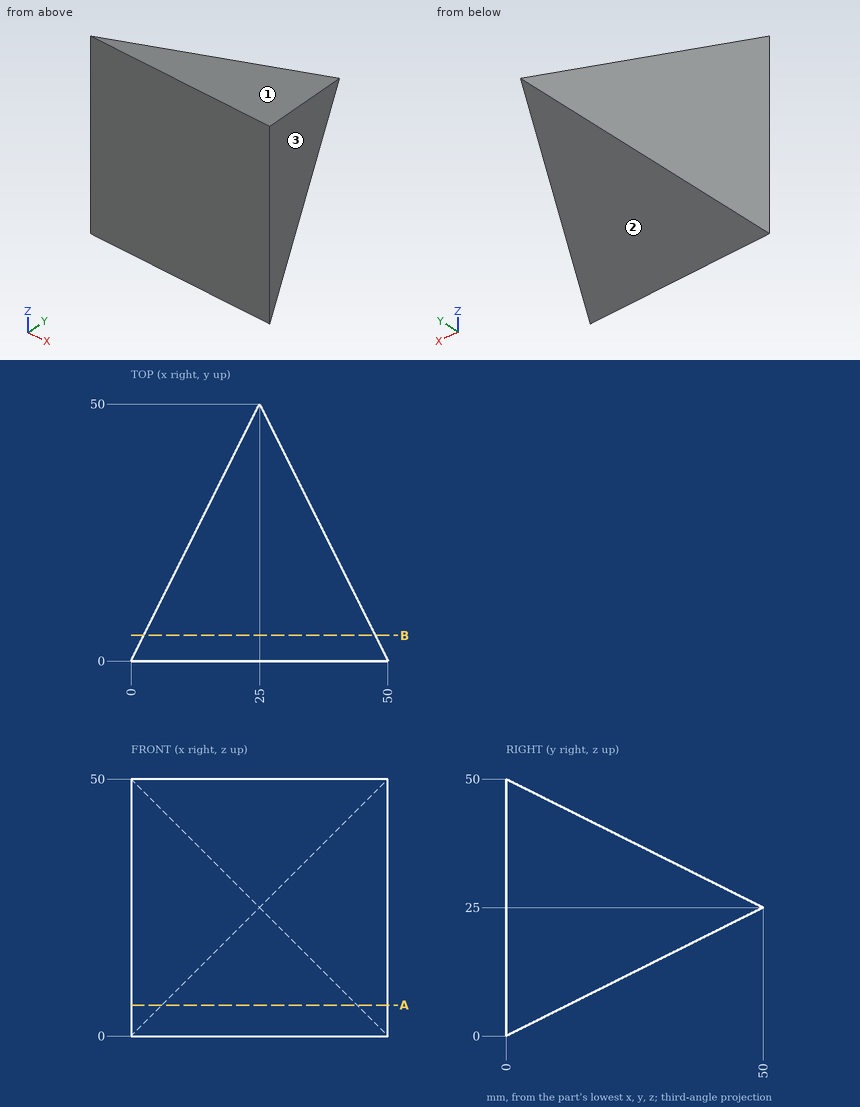
Study the drawing (mm; zero at the part's minimum x, y, z) and answer. Coordinates: 2 decimals unless noted, no trailing zeros. Loops run counter-clockwise (first coordinate to the right, second up) from the corner with the lowest first, then second, coordinate; pieces in that order, holes last. Notation, with made-up numbers: (67, 0) -> (113, 0) arc R29 ccw to (113, 37) -> close; hole circle Ø6 at (24.25, 59.25). An arc over 180 degrees is marked (long way). Write item = value, one per line. Start each with the question number.
1) The mould has two halves that part along Z. Classify the marked faces 1, 2 and 3: pulls with the +Z half, pulls with the -Z half, needs draft (parallel to the pull), parting line crosses it, or undercut.
2) Given P1, Ø1, axis at y = 25, z = 13.5, coming from the -X side; P2, Ø10, axis at y = 17.5, z = 34.5, coming from the -X side; P3, Ø4, axis at y = 7, z = 20.5, coming from the +X side, each flat-ended and moving along its own axis, determine where each tip first touches the part or whether it passes through.
3) Find the intervals of material crossed by L1, parallel to X at y = 45.5, z = 27; L2, parallel to Y at x = 38, z = 42; L3, parallel to Y at x = 47, z = 31.5, in increasing order. Write a range as from..to.
4) The part is cut by section B-B, the plane y = 5. Determine the outline of the cut face in (x, z), plus the area to 4 significant figures.
5) The part is cut by section A-A, the plane z = 6. Determine the outline of the cut face in (x, y).
Result:
q1.face_1 = pulls with the +Z half
q1.face_2 = pulls with the -Z half
q1.face_3 = needs draft
q2.P1 = 12.25
q2.P2 = 6.25
q2.P3 = 47.5
q3.L1 = 22.75..27.25
q3.L2 = 0..16
q3.L3 = 0..6
q4.outline = (2.5, 2.5) -> (47.5, 2.5) -> (47.5, 47.5) -> (2.5, 47.5) -> close
q4.area = 2,025 mm²
q5.outline = (0, 0) -> (50, 0) -> (44, 12) -> (6, 12) -> close
